Could you check a few things on this model? Use its own coordinates, in mm. A direction names the side the tool comes from. Coordinates: 2 decimals unless noted, no trailing zeros. Loops run counter-clockwise (first coordinate to the right, second up) from the corner with the lowest first, then second, coordinate; pieces in that order, holes last. Notation, with made-up numbers: M -3.5,41 L 51.5,41 A19 ccw 51.5,58 Z; hole C 19.5,53 d3. An arc over 180 degrees is marked long. Write each question's results on one line, items separated by ' | '.
```python
from build123d import *

# Parameters (mm, degrees)
BOSS_EXTRUDE1_OUTLINE_R = 1.5875
BOSS_EXTRUDE1_OUTLINE_W = 1.5875
BOSS_EXTRUDE1_OUTLINE_H = 6.35
BOSS_EXTRUDE1_DEPTH     = 1.5875
FILLET1_R               = 3.175


# Read off the part's stored shape, not the designer's step: Boss-Extrude1
with BuildPart() as part:
    # Boss-Extrude1 outline → Boss-Extrude1 (new body)
    with BuildSketch(Plane.XY):
        with BuildLine():
            ThreePointArc((142.057282468, 6.553787305), (156.214269946, 11.485509293), (142.057282468, 16.417231281))
            ThreePointArc((142.057282468, 16.417231281), (140.813384973, 15.816075679), (139.569487477, 16.417231281))
            ThreePointArc((139.569487477, 16.417231281), (132.172803886, 19.335230024), (125.957459481, 14.375881403))
            ThreePointArc((125.957459481, 14.375881403), (124.82332848, 13.404258866), (123.384428498, 13.804096739))
            ThreePointArc((123.384428498, 13.804096739), (116.794815058, 15.913313858), (111.053922915, 12.051454261))
            ThreePointArc((111.053922915, 12.051454261), (108.094534878, 12.329767665), (105.240273774, 11.499930657))
            Line((105.240273774, 11.499930657), (91.492120489, 3.562430657))
            ThreePointArc((91.492120489, 3.562430657), (90.329989832, -0.7747), (94.667120489, -1.936830657))
            Line((94.667120489, -1.936830657), (101.318750253, 1.903489577))
            ThreePointArc((101.318750253, 1.903489577), (102.647339692, -0.532407494), (104.733149805, -2.3622))
            Line((104.733149805, -2.3622), (112.955202512, -2.3622))
            ThreePointArc((112.955202512, -2.3622), (114.503673459, -1.137682555), (115.702067342, 0.431093193))
            ThreePointArc((115.702067342, 0.431093193), (121.421294864, 0.935289323), (125.304354616, 5.164429205))
            ThreePointArc((125.304354616, 5.164429205), (126.438485618, 6.136051741), (127.8773856, 5.736213868))
            ThreePointArc((127.8773856, 5.736213868), (133.903679898, 3.567343797), (139.569487477, 6.553787305))
            ThreePointArc((139.569487477, 6.553787305), (140.813384973, 7.154942907), (142.057282468, 6.553787305))
        make_face()
        with Locations((95.169339789, 2.0193)):
            Circle(BOSS_EXTRUDE1_OUTLINE_R, mode=Mode.SUBTRACT)
        with Locations((101.988423818, 5.9563)):
            Circle(BOSS_EXTRUDE1_OUTLINE_R, mode=Mode.SUBTRACT)
        Polygon((110.516780309, 1.614730068), (108.996231081, 1.158565299), (107.171572008, 7.24076221), (108.692121236, 7.696926979), align=None, mode=Mode.SUBTRACT)
        Polygon((118.248573702, 11.310144159), (119.146599315, 5.023964874), (117.575054493, 4.799458471), (116.677028881, 11.085637756), align=None, mode=Mode.SUBTRACT)
        with Locations((133.35, 11.485509293)):
            Rectangle(BOSS_EXTRUDE1_OUTLINE_W, BOSS_EXTRUDE1_OUTLINE_H, mode=Mode.SUBTRACT)
        Polygon((149.311693327, 14.590279439), (148.82467056, 8.258983456), (147.241846564, 8.380739148), (147.728869332, 14.71203513), align=None, mode=Mode.SUBTRACT)
    extrude(amount=BOSS_EXTRUDE1_DEPTH)

    # Fillet1
    fillet1_edges = [part.edges().sort_by_distance(p)[0] for p in [
        (115.702067342, 0.431093193, 0.79375),
        (112.955202512, -2.3622, 0.79375),
        (104.733149805, -2.3622, 0.79375),
        (101.318750253, 1.903489577, 0.79375),
        (111.053922915, 12.051454261, 0.79375),
    ]]
    fillet(fillet1_edges, radius=FILLET1_R)


solid = part.part
```
(1) Will these pins go through, and if not, where does the flat tip stop? P1, Ø8, axis at x = 146, y = 6, coming from the -Z side; P2, Ø0.5, axis at y = 10, z = 0.5, coming from the -X side.
Reported:
P1: stops at z = 0 | P2: stops at x = 102.21
(2) If we mould it in two halves opening along Y, with no side actions, what happens to faces 4 (the cylindrical face through (100.749, 0.657, 0.805)), 5 (the cylindrical face through (117.7, 15.99, 0.78)), 6 (the flat face through (109.59, 4.7, 0.78)), 7 (the flat face through (134.144, 11, 1))? For each: released by +Y, released by -Y, zero draft, split by the parting line, or undercut.
Reported:
face 4: released by -Y | face 5: released by +Y | face 6: undercut | face 7: undercut
(3) Which directions (+Z, -Z, +X, -X, +Y, -Y) give clear straight access to the entire face, cutting with the end or side of a thin tool? Please do faces 1 (the flat face through (96.57, -0.84, 0.78)), 2 (the flat face through (109, -2.362, 1)), 3 (the flat face through (148.04, 8.32, 0.78)).
Reported:
face 1: +Z, -Z, -Y | face 2: +Z, -Z, +X, -X, -Y | face 3: +Z, -Z
(4) Imagine slicing it at D-D, the plane x = 97.5. List the corners of the cut face in (y, z) for me.
Reported:
outline: M -0.3,0 L 7.03,0 L 7.03,1.59 L -0.3,1.59 Z
(5) Imagine slicing it at A-A, the plane y = 17. List the corners of the cut face in (x, z) for me, and give its area (3 significant figures).
Reported:
outline: M 127.64,0 L 139.06,0 L 139.06,1.59 L 127.64,1.59 Z; M 142.57,0 L 153.99,0 L 153.99,1.59 L 142.57,1.59 Z | area: 36.3 mm2
(6) Imagine slicing it at B-B, the plane z = 0.55. State how many separate pieces and enclosed holes the cut face has, and give its area (3 significant figures).
Reported:
separate pieces: 1 | enclosed holes: 6 | area: 759 mm2
(7) Imagine slicing it at C-C, the plane x = 146. List the corners of the cut face in (y, z) for me, and give its area (3 significant figures).
Reported:
outline: M 3.88,0 L 19.09,0 L 19.09,1.59 L 3.88,1.59 Z | area: 24.1 mm2
(8) Please list where these lines run through material, in increasing order: probe 1 along X at (y, z) = (2.25, 0.25); probe 2 along X at (y, z) = (14.5, 0.55); probe 3 along X at (y, z) = (11.5, 1). Write a range as from..to.
Reported:
probe 1: x = 90.25..93.6, 96.74..108.67, 110.33..123.33 | probe 2: x = 113.28..122.54, 126.01..132.56, 134.14..147.71, 149.3..155.62 | probe 3: x = 105.24..132.56, 134.14..147.48, 149.07..156.21
